```python
from build123d import *

# Parameters (mm, degrees)
F2_DEPTH = 1
F3_DEPTH = 1
F4_R     = 0.75
F5_DEPTH = 25.4


with BuildPart() as f2:
    # F0 (on Front) → F2 (new body)
    with BuildSketch(Plane.XZ):
        Polygon((-54.62, 0), (0, 0), (0, 29.45), align=None)
        Polygon((0, 29.45), (0, 0), (54.62, 0), align=None)
    extrude(amount=-F2_DEPTH)

    # F1 (on Right) → F3 (join)
    with BuildSketch(Plane.YZ):
        Polygon((0, 14.36), (0, 0), (26.66, 0), align=None)
        Polygon((-26.66, 0), (0, 0), (0, 14.36), align=None)
    extrude(amount=F3_DEPTH)

    # F4 (on Top) → F5 (join)
    with BuildSketch(Plane.XY):
        with Locations((0.486322, 0.526076)):
            Circle(F4_R)
    extrude(amount=-F5_DEPTH)


solid = f2.part
```
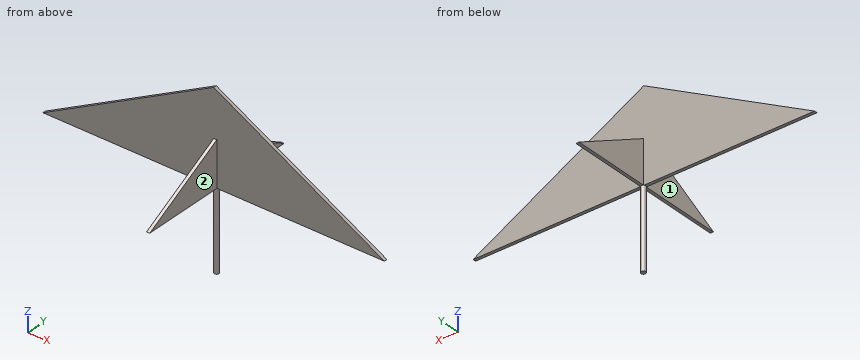
Input: part model. Units: mm. Frame: model coordinates. Face numbers are marked on the shaded views. A direction names the side the tool comes from. Round coordinates to 2 decimals unless told otherwise and drop trailing zeros. Loops run counter-clockwise (first coordinate to the right, second up) from the corner with the lowest first, then second, coordinate; pieces in that order, holes last. Notation, with made-up numbers: (-25.5, -35.75) -> (-2.5, -35.75) arc R18 cw to (-2.5, -10.75) -> close; hole circle Ø3 at (-27, 25). An arc over 180 degrees is marked (long way). Use one line per item in the form item = value. Start each with the question number.
Item 1: Section query B-B on x = 4.5. Return the cut outline in (y, z), then the cut area to 3 significant figures.
Item 2: Contact query for flat-ended pins moving along their axis: pin 1 Ø1.1 at (x, y) = (-30, 0.5) entering from -Z; pin 2 Ø11.5 at (y, z) = (-14, 10) entering from +X; pin 3 Ø14.5 at (x, z) = (-7.5, 12) entering from +Y. Output: stop coordinate, or through.
Item 3: Material intervals for L1, parallel to Y at x = 0.5, z = -10; L2, parallel to X at y = 12.5, z = 3, sorted ascending. Write a range as from..to.
Item 4: Section query D-D on z = -5. Return the cut outline in (x, y), then the cut area to 3 significant figures.
Item 5: Section query A-A on z = 6.5. Return the cut outline in (x, y), then the cut area to 3 significant figures.
Item 6: Set-up query: the marked faces 1 and 2. Return all of +Z, -Z, +X, -X, +Y, -Y with unobstructed straight access to the full face (end or side cutting, diameter ignored); none if empty.
Item 7: Section query C-C on y = 6. Return the cut outline in (x, z), then the cut area to 3 significant figures.
Ans:
q1.outline = (0, 0) -> (1, 0) -> (1, 27.02) -> (0, 27.02) -> close
q1.area = 27.0 mm^2
q2.pin_1 = 0
q2.pin_2 = 1
q2.pin_3 = 1
q3.L1 = -0.22..1.28
q3.L2 = 0..1
q4.outline = circle Ø1.5 at (0.49, 0.53)
q4.area = 1.77 mm^2
q5.outline = (-42.56, 0) -> (0, 0) -> (0, -14.59) -> (1, -14.59) -> (1, 0) -> (42.56, 0) -> (42.56, 1) -> (1, 1) -> (1, 14.59) -> (0, 14.59) -> (0, 1) -> (-42.56, 1) -> close
q5.area = 113 mm^2
q6.face_1 = +Z, -Z, -X, -Y
q6.face_2 = +Z, -Z, +X, -Y
q7.outline = (0, 0) -> (1, 0) -> (1, 11.13) -> (0, 11.13) -> close
q7.area = 11.1 mm^2
